Check sheet for the modelled part. Datum: model origin and axes. Units: mm. A direction names the side the tool comes from. Coordinates: 2 decimals unless noted, no trailing zeros. Order: outer loops, then holes, each group sorted by start corner. A loop starts at its lowest first (then second) coordinate and runs counter-clockwise, first axis right, second up.
1. Gauge pin test, flat ends, axial feed: pin 1 Ø4 at (x, y) = (9, -4) entering from +Z; pin 2 Ø2.5 at (y, z) = (-4, 39) entering from +X; pin 3 Ø2.5 at (x, y) = (8, -4.5) entering from -Z. Record the tip position at first contact, or that the pin passes through.
2. Set-up check for faces 1 (the flat face through (40, -4, 110)), 2 (the flat face through (44, -4, -105.25)), 3 (the flat face through (40, -4, 60)): record each of +Z, -Z, +X, -X, +Y, -Y from which the full face is reachable in a straight line by a thin tool's end or side.
3. Cross-section at D-D (x = 21). Enter the section's corners in (y, z).
4. Cross-section at A-A (y = -2.5). Enter the section's corners in (x, z), then the cut area to 3 significant figures.
5. Cross-section at C-C (z = -17). Enter the section's corners in (x, y).
6. Thickness scan on line 1 (Z direction, x = 20, y = -4.5); line 2 (Z direction, x = 15, y = -0.75); line 3 (X direction, y = -5.5, z = -24). Record the ranges inside material, lowest first.
7. Cross-section at B-B (x = 2). Enter the section's corners in (y, z).
```python
from build123d import *

# Parameters (mm, degrees)
F0_W     = 8
F0_H     = 40
F1_DEPTH = 8


# Not quite as in the source:
# - ends of sketch curves that miss each other by under 0.0002 mm in the source are joined


with BuildPart() as f1:
    # F0 (on Front) → F1 (new body)
    with BuildSketch(Plane.XZ):
        with Locations((44, 85.25)):
            Rectangle(F0_W, F0_H)
        with Locations((44, -85.25)):
            Rectangle(F0_W, F0_H)
        with BuildLine():
            Line((30, -45.25), (-29.7788833363, -45.25))
            ThreePointArc((-29.7788833363, -45.25), (-9.3545962046, -94.6694618691), (40, -115.25))
            Line((40, -115.25), (40, -105.25))
            Line((40, -105.25), (40, -65.25))
            Line((40, -65.25), (40, -55.25))
            ThreePointArc((40, -55.25), (32.9289321881, -52.3210678119), (30, -45.25))
        make_face()
        with BuildLine():
            ThreePointArc((40, 115.25), (-9.4974751888, 94.7474741773), (-30, 45.2499985695))
            Line((-30, 45.2499985695), (30, 45.25))
            ThreePointArc((30, 45.25), (32.9289321881, 52.3210678119), (40, 55.25))
            Line((40, 55.25), (40, 65.25))
            Line((40, 65.25), (40, 105.25))
            Line((40, 105.25), (40, 115.25))
        make_face()
        Polygon((-30, 45.25), (-30, -45.25), (-29.7788833363, -45.25), (30, -45.25), (30, -35.25), (0, -35.25), (0, -27.25), (30, -27.25), (30, 12.75), (0, 12.75), (0, 20.75), (30, 20.75), (30, 45.25), align=None)
    extrude(amount=F1_DEPTH)


solid = f1.part
```
Data:
1. pin 1: stops at z = 108.96
1. pin 2: stops at x = 30
1. pin 3: stops at z = -108.03
2. face 1: +Z, +X, +Y, -Y
2. face 2: -Z, +X, +Y, -Y
2. face 3: +X, +Y, -Y
3. outline: (-8, -112.56) - (0, -112.56) - (0, -35.25) - (-8, -35.25) - close; (-8, -27.25) - (0, -27.25) - (0, 12.75) - (-8, 12.75) - close; (-8, 20.75) - (0, 20.75) - (0, 112.62) - (-8, 112.62) - close
4. outline: (-30, -45.25) - (-29.78, -45.25) arc R70 ccw to (40, -115.25) - (40, -105.25) - (48, -105.25) - (48, -65.25) - (40, -65.25) - (40, -55.25) arc R10 cw to (30, -45.25) - (30, -35.25) - (0, -35.25) - (0, -27.25) - (30, -27.25) - (30, 12.75) - (0, 12.75) - (0, 20.75) - (30, 20.75) - (30, 45.25) arc R10 cw to (40, 55.25) - (40, 65.25) - (48, 65.25) - (48, 105.25) - (40, 105.25) - (40, 115.25) arc R70 ccw to (-30, 45.25) - close
4. area: 13,100 mm2
5. outline: (-30, -8) - (30, -8) - (30, 0) - (-30, 0) - close
6. line 1: z = -112.27 to -35.25, -27.25 to 12.75, 20.75 to 112.33
6. line 2: z = -110.55 to -35.25, -27.25 to 12.75, 20.75 to 110.63
6. line 3: x = -30 to 30
7. outline: (-8, -103.89) - (0, -103.89) - (0, -35.25) - (-8, -35.25) - close; (-8, -27.25) - (0, -27.25) - (0, 12.75) - (-8, 12.75) - close; (-8, 20.75) - (0, 20.75) - (0, 104.04) - (-8, 104.04) - close
